```python
from build123d import *

# Parameters (mm, degrees)
SKETCH1_R                = 3.4
BOSS_EXTRUDE1_DEPTH      = 7
SKETCH4_R                = 5
BOSS_EXTRUDE2_DEPTH      = 1
SKETCH5_R                = 4
BOSS_EXTRUDE3_DEPTH      = 5
CUT_EXTRUDE1_DEPTH       = 3
FILLET1_R                = 0.5
CIRPATTERN1_COUNT        = 2
CIRPATTERN1_ANGLE        = 90
FILLET1_OF_CIRPATTERN1_R = 0.5
SKETCH7_W                = 13.377916116
SKETCH7_H                = 10.003544581
SKETCH7_W_2              = 13.109283262
SKETCH7_H_2              = 10.863169713
CUT_EXTRUDE2_DEPTH       = 58.393379409


# Read off the part's stored shape, not the designer's step: Imported1
with BuildPart() as part:
    # Sketch1 → Boss-Extrude1 (new body)
    with BuildSketch(Plane(origin=(0, 7, 0), x_dir=(1, 0, 0), z_dir=(0, 1, 0))):
        with BuildLine():
            Line((-25, 20), (-25, -20))
            ThreePointArc((-25, -20), (-23.535533906, -23.535533906), (-20, -25))
            Line((-20, -25), (20, -25))
            ThreePointArc((20, -25), (23.535533906, -23.535533906), (25, -20))
            Line((25, -20), (25, 20))
            ThreePointArc((25, 20), (23.535533906, 23.535533906), (20, 25))
            Line((20, 25), (-20, 25))
            ThreePointArc((-20, 25), (-23.535533906, 23.535533906), (-25, 20))
        make_face()
        with Locations(Location((0, 0, 0), (0, 0, 270))):
            Circle(SKETCH1_R, mode=Mode.SUBTRACT)
    extrude(amount=-BOSS_EXTRUDE1_DEPTH)

    # Sketch4 → Boss-Extrude2 (add)
    with BuildSketch(Plane(origin=(0, 7, 0), x_dir=(1, 0, 0), z_dir=(0, 1, 0))):
        with Locations(Location((0, 14.2, 0), (0, 0, 270))):
            Circle(SKETCH4_R)
        with Locations(Location((0, -14.2, 0), (0, 0, 270))):
            Circle(SKETCH4_R)
    boss_extrude2 = extrude(amount=BOSS_EXTRUDE2_DEPTH)

    # Sketch5 → Boss-Extrude3 (add)
    with BuildSketch(Plane(origin=(0, 8, 0), x_dir=(1, 0, 0), z_dir=(0, 1, 0))):
        with Locations(Location((0, 14.2, 0), (0, 0, 270))):
            Circle(SKETCH5_R)
        with Locations(Location((0, -14.2, 0), (0, 0, 270))):
            Circle(SKETCH5_R)
    boss_extrude3 = extrude(amount=BOSS_EXTRUDE3_DEPTH)

    # Sketch6 → Cut-Extrude1 (cut)
    with BuildSketch(Plane(origin=(0, 13, 0), x_dir=(1, 0, 0), z_dir=(0, 1, 0))):
        Polygon((0, 16.798076211), (-2.25, 15.499038106), (-2.25, 12.900961894), (0, 11.601923789), (2.25, 12.900961894), (2.25, 15.499038106), align=None)
        Polygon((0, -11.601923789), (-2.25, -12.900961894), (-2.25, -15.499038106), (0, -16.798076211), (2.25, -15.499038106), (2.25, -12.900961894), align=None)
    cut_extrude1 = extrude(amount=-CUT_EXTRUDE1_DEPTH, mode=Mode.SUBTRACT)

    # Fillet1
    fillet1_edges = [part.edges().sort_by_distance(p)[0] for p in [
        (0, 13, -18.2),
        (0, 13, 10.2),
    ]]
    fillet(fillet1_edges, radius=FILLET1_R)

    # CirPattern1: Boss-Extrude2, Boss-Extrude3, Cut-Extrude1 ×2 about axis
    cirpattern1_axis = Axis((0, 0, 0), (0, -1, 0))
    add([boss_extrude2.rotate(cirpattern1_axis, i * CIRPATTERN1_ANGLE / (CIRPATTERN1_COUNT - 1)) for i in range(1, CIRPATTERN1_COUNT)])
    add([boss_extrude3.rotate(cirpattern1_axis, i * CIRPATTERN1_ANGLE / (CIRPATTERN1_COUNT - 1)) for i in range(1, CIRPATTERN1_COUNT)])
    add([cut_extrude1.rotate(cirpattern1_axis, i * CIRPATTERN1_ANGLE / (CIRPATTERN1_COUNT - 1)) for i in range(1, CIRPATTERN1_COUNT)], mode=Mode.SUBTRACT)

    # Fillet1 of CirPattern1
    fillet1_of_cirpattern1_edges = [part.edges().sort_by_distance(p)[0] for p in [
        (18.2, 13, 0),
        (-10.2, 13, 0),
    ]]
    fillet(fillet1_of_cirpattern1_edges, radius=FILLET1_OF_CIRPATTERN1_R)

    # Sketch7 → Cut-Extrude2 (cut, through all)
    with BuildSketch(Plane(origin=(25, 0, 0), x_dir=(0, 0, -1), z_dir=(1, 0, 0))):
        with Locations((14.04949825, 12.00177229)):
            Rectangle(SKETCH7_W, SKETCH7_H)
        with Locations((-13.592822399, 12.431584857)):
            Rectangle(SKETCH7_W_2, SKETCH7_H_2)
    extrude(amount=-CUT_EXTRUDE2_DEPTH, mode=Mode.SUBTRACT)


solid = part.part
```
Geometry check sheet. Reference: the model listing, model coordinates, mm. A direction names the side the tool comes from. Give positions to 0.01 mm unless a question says otherwise; leave off trailing zeros. Write each loop counter-clockwise with the first axis right and the second up, starting at its lowest first coordinate (ties: lowest second). Pieces come first, ordered by that corner, then holes. Notation, with made-up numbers: (-28, -10) -> (-18, -10) arc R16 ccw to (-18, 1) -> close; hole circle Ø1 at (56, 66). An arc over 180 degrees is marked (long way). One line per question, with ' | ' between items.
Item 1: Draft check along X on faces 3 (the cylindrical face through (18.196, 10.218, 0.176)), 4 (the flat face through (12, 13, -1)), 5 (the flat face through (-12.242, 11.521, -1.109)), 6 (the flat face through (25, 4, 0)). Enter one of: released by +X, released by -X, zero draft, split by the parting line, or undercut.
Determined:
face 3: undercut | face 4: zero draft | face 5: undercut | face 6: released by +X
Item 2: Sectioned sample at A-A, the plane y = 11.5. Record the boundary of the cut face in (x, z), plus the area to 3 significant figures.
Determined:
outline: circle Ø8 at (-14.2, 0); circle Ø8 at (14.2, 0); hole (-16.8, 0) -> (-15.5, -2.25) -> (-12.9, -2.25) -> (-11.6, 0) -> (-12.9, 2.25) -> (-15.5, 2.25) -> close; hole (11.6, 0) -> (12.9, -2.25) -> (15.5, -2.25) -> (16.8, 0) -> (15.5, 2.25) -> (12.9, 2.25) -> close | area: 65.5 mm^2
Item 3: Sectioned sample at D-D, the plane x = -14.2. Record the boundary of the cut face in (y, z).
Determined:
outline: (0, -25) -> (7, -25) -> (7, -5) -> (8, -5) -> (8, -4) -> (12.5, -4) arc R0.5 ccw to (13, -3.5) -> (13, -2.25) -> (10, -2.25) -> (10, 2.25) -> (13, 2.25) -> (13, 3.5) arc R0.5 ccw to (12.5, 4) -> (8, 4) -> (8, 5) -> (7, 5) -> (7, 25) -> (0, 25) -> close
Item 4: Depth check by flat-ended pin: pin 1 (25 mm diameter, centred on x = -3, z = 11.5, fed in from +Y); pin 2 (1.3 mm diameter, centred on x = -14, y = 11, fed in from -Z); pin 3 (2 mm diameter, centred on x = 15, y = 11, fed in from +Z). Enter the tip coordinate at first touch or a pass-through.
Determined:
pin 1: y = 13 | pin 2: z = -4 | pin 3: z = 4
Item 5: Sectioned sample at B-B, the plane y = 1.5. Record the boundary of the cut face in (x, z).
Determined:
outline: (-25, -20) arc R5 ccw to (-20, -25) -> (20, -25) arc R5 ccw to (25, -20) -> (25, 20) arc R5 ccw to (20, 25) -> (-20, 25) arc R5 ccw to (-25, 20) -> close; hole circle Ø6.8 at (0, 0)
Item 6: Access from +Z, -Z, +X, -X, +Y, -Y to the whole of each face (thin tool, end or side, straight path). Record for faces 1 (the flat face through (14, 10, 0)), 2 (the flat face through (0, 4, -25)).
Determined:
face 1: +Y | face 2: -Z, +X, -X, +Y, -Y
Item 7: Sectioned sample at C-C, the plane x = 0. Record the boundary of the cut face in (y, z).
Determined:
outline: (0, -25) -> (7, -25) -> (7, -3.4) -> (0, -3.4) -> close; (0, 3.4) -> (7, 3.4) -> (7, 25) -> (0, 25) -> close
Item 8: Scan lines: line 1 along X through (y, z) = (5, 0); line 2 along Y through (x, z) = (-7, -20); line 3 along X through (y, z) = (11.75, 2). Record each from-to range of solid material in increasing order.
Determined:
line 1: -25 to -3.4, 3.4 to 25 | line 2: 0 to 7 | line 3: -17.66 to -15.64, -12.76 to -10.74, 10.74 to 12.76, 15.64 to 17.66
